The model under review builds one solid part; all positions refer to its coordinate system, in mm. Face numbers are marked on the shaded views. A direction names the side the tool comes from. Round coordinates to 2 decimals unless told otherwise and drop trailing zeros. Order: outer loops, then holes, each group sorted by start corner. A loop starts at its lowest first (then second) coordinate and runs counter-clockwise, first axis right, second up.
```python
from build123d import *

# Parameters (mm, degrees)
SKETCH_2_R           = 7
EXTRUDE_1_DEPTH      = 15
EXTRUDE_1_DEPTH_BACK = 5


with BuildPart() as part:
    # Эскиз1 → Повернуть2 (revolve)
    with BuildSketch(Plane.XY):
        Polygon((0, 0), (5.740181269, 0), (8.157099698, 50), (15, 50), (15, 62.386706949), (11.480362538, 62.386706949), (11.480362538, 69.637462236), (21.148036254, 69.637462236), (21.148036254, 84.743202417), (15, 84.743202417), (10, 170), (0, 170), align=None)
    revolve(axis=Axis((0, 0, 0), (0, 1, 0)))

    # Эскиз2 → Бобышка-Вытянуть1 (add, two sides)
    with BuildSketch(Plane(origin=(21.148036254, 0, 0), x_dir=(0, 0, -1), z_dir=(1, 0, 0))) as extrude_1_sk:
        with Locations((0, 77.29820462)):
            Circle(SKETCH_2_R)
    extrude(amount=EXTRUDE_1_DEPTH)
    extrude(extrude_1_sk.sketch, amount=-EXTRUDE_1_DEPTH_BACK)

    # Эскиз3 → Повернуть3 (revolve)
    with BuildSketch(Plane(origin=(0, 0, 0), x_dir=(0, 0, -1), z_dir=(1, 0, 0))):
        Polygon((-49.069170568, 77), (-49.069170568, 86.826198905), (-43.352373997, 86.826198905), (-29.695582188, 81.913099452), (-29.695582188, 80.156602905), (-20.167587903, 80.156602905), (-20.167587903, 77), align=None)
    revolve(axis=Axis((0, 77, 70.030757994), (0, 0, -1)))


solid = part.part
```
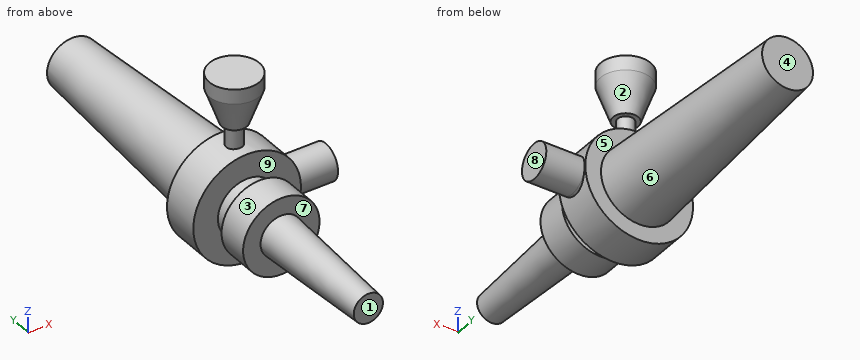
(1) For the marked faces 1, 2, 3, 4 and 5, list the 3-axis set-ups (+Z, -Z, +X, -X, +Y, -Y) from which the entire face can be reached by the end or side of a thin tool; tool diameter is ignored.
Data:
face 1: +Z, -Z, +X, -X, -Y
face 2: none
face 3: -Y
face 4: +Z, -Z, +X, -X, +Y
face 5: +Y
(2) Consider section C-C (y = 13). Write out the cut boundary in (x, z).
Data:
outline: circle Ø12.74 at (0, 0)
(3) Draft analysis for pull direction Y (two halves, no side actions). For the marked faces 6, 7, 8 and 9, state which applies: pulls with the +Y half, pulls with the -Y half, needs draft (parallel to the pull), parting line crosses it, or undercut.
Data:
face 6: pulls with the +Y half
face 7: pulls with the -Y half
face 8: needs draft
face 9: undercut
(4) Consider section B-B (z = 27.5). Write out the cut boundary in (x, y), and give its area (3 significant figures).
Data:
outline: circle Ø6.31 at (0, 77)
area: 31.3 mm2
(5) To check wall thickness, follow probe 1 along Y at (x, z) = (8, -15); probe 2 along Z at (x, y) = (0, 58.5); probe 3 along Y at (x, z) = (-1, 31.5). State the ranges of each line that lie inside material, in increasing order.
Data:
probe 1: y = 69.64 to 84.74
probe 2: z = -15 to 15
probe 3: y = 71.53 to 82.47
(6) Insertion check: pin 1 (10 mm diameter, centred on x = -9.5, z = 10, fed in from +Y); pin 2 (12 mm diameter, centred on x = 1, y = 30.5, fed in from -Z); pin 3 (2 mm diameter, centred on x = 5, z = 33, fed in from -Y); pin 4 (11 mm diameter, centred on x = -1, y = 76.5, fed in from -Z). Each pin has a flat end and moves straight along its axis. Give the tip position at first contact, or say it passes through.
Data:
pin 1: stops at y = 170
pin 2: stops at z = -7.5
pin 3: stops at y = 72.27
pin 4: stops at z = -21.15
